```python
from build123d import *

# Parameters (mm, degrees)
SKETCH1_R           = 82.5
BOSS_EXTRUDE1_DEPTH = 13
SKETCH2_R           = 30
CUT_EXTRUDE1_DEPTH  = 118.394633608
SKETCH3_R           = 6.451717482
CUT_EXTRUDE2_DEPTH  = 7.921699
CIRPATTERN1_START   = 5.0783014
CIRPATTERN1_DEPTH   = 7.9216986


# Read off the part's stored shape, not the designer's step: CirPattern1
with BuildPart() as part:
    # Sketch1 → Boss-Extrude1 (new body)
    with BuildSketch(Plane(origin=(0, 0, 0), x_dir=(1, 0, 0), z_dir=(0, 1, 0))):
        with Locations(Location((0, 0, 0), (0, 0, 90))):
            Circle(SKETCH1_R)
    extrude(amount=BOSS_EXTRUDE1_DEPTH)

    # Sketch2 → Cut-Extrude1 (cut, through all)
    with BuildSketch(Plane(origin=(0, 0, 0), x_dir=(1, 0, 0), z_dir=(0, 1, 0))):
        with Locations(Location((0, 0, 0), (0, 0, 90))):
            Circle(SKETCH2_R)
    extrude(amount=CUT_EXTRUDE1_DEPTH, mode=Mode.SUBTRACT)

    # Sketch3 → Cut-Extrude2 (cut)
    with BuildSketch(Plane(origin=(0, 13, 0), x_dir=(1, 0, 0), z_dir=(0, 1, 0))):
        with Locations((-29.738341357, 0)):
            Circle(SKETCH3_R)
    extrude(amount=-CUT_EXTRUDE2_DEPTH, mode=Mode.SUBTRACT)

    # CirPattern1 outline → CirPattern1 (cut)
    with BuildSketch(Plane(origin=(0, 0, 0), x_dir=(1, 0, 0), z_dir=(0, 1, 0)).offset(CIRPATTERN1_START)):
        with BuildLine():
            ThreePointArc((-9.076134205, -28.594121562), (-15, -25.980762114), (-20.225168569, -22.157223571))
            ThreePointArc((-20.225168569, -22.157223571), (-18.095029419, -31.341510319), (-9.076134205, -28.594121562))
        make_face()
        with BuildLine():
            ThreePointArc((-9.076134205, 28.594121562), (-18.095029419, 31.341510319), (-20.225168569, 22.157223571))
            ThreePointArc((-20.225168569, 22.157223571), (-15, 25.980762114), (-9.076134205, 28.594121562))
        make_face()
        with BuildLine():
            ThreePointArc((20.225168569, -22.157223571), (15, -25.980762114), (9.076134205, -28.594121562))
            ThreePointArc((9.076134205, -28.594121562), (18.095029419, -31.341510319), (20.225168569, -22.157223571))
        make_face()
        with BuildLine():
            ThreePointArc((20.225168569, 22.157223571), (18.095029419, 31.341510319), (9.076134205, 28.594121562))
            ThreePointArc((9.076134205, 28.594121562), (15, 25.980762114), (20.225168569, 22.157223571))
        make_face()
        with BuildLine():
            ThreePointArc((29.301302774, 6.436897991), (30, 0), (29.301302774, -6.436897991))
            ThreePointArc((29.301302774, -6.436897991), (36.190058839, 0), (29.301302774, 6.436897991))
        make_face()
    extrude(amount=CIRPATTERN1_DEPTH, mode=Mode.SUBTRACT)


solid = part.part
```
Could you check a few things on this model? Use its own coordinates, in mm. A direction names the side the tool comes from. Round coordinates to 2 decimals unless told otherwise and drop trailing zeros. Write each loop counter-clockwise with the first axis right and the second up, starting at its lowest first coordinate (ties: lowest second). Pieces come first, ordered by that corner, then holes. Notation, with made-up numbers: M 37.5,51.5 L 41.5,51.5 A16 cw 41.5,65.5 Z; hole C 65,-18.5 d4. An arc over 180 degrees is marked long. Answer in a Markdown table with one row per item. Add a question column.
Q1. Imagine slicing it at D-D (z = 48). Please give me the cut outline in (x, y).
Q2. Will these pins go through, and if not, where does the flat tip stop? pin 1 Ø1.5 at (y, z) = (5, -10.5) entering from +X; pin 2 Ø1 at (y, z) = (10, 42) entering from +X; pin 3 Ø8 at (x, z) = (-16.5, -27) entering from +Y.
Q3. If we mould it in two halves opening along X, with no side actions, what happens to faces 3 (the cylindrical face through (80.54, 6.41, 17.88)), 4 (the flat face through (-1, 0, -36)), 5 (the flat face through (-17, 5.078, 28))? For each: +X half, -X half, draft (parallel to the pull), parting line (faces both ways), or undercut.
Q4. Imagine slicing it at A-A (z = 0). Please give me the cut outline in (x, y).
Q5. If I drill on line 1 (X direction, y = 5, z = 0); line 2 (Z direction, x = 1, y = 8); line 3 (X direction, y = 9, z = 27), over which ranges is the centre line in solid material (lowest first)? Write a range as from..to.
Q6. On a 3-axis mill with a long thin cutter (end or side, diameter ignored), from which of +Z, -Z, +X, -X, +Y, -Y can I reach the whole of each face in a straight line? I mean faces 1 (the flat face through (-1, 13, -36)), 2 (the cylindrical face through (18.222, 8.984, -31.266)). Say none if no direction works.
Q7. Imagine slicing it at C-C (y = 7.75). Please give me the cut outline in (x, z), then the cut area to 3 significant figures.
Q8. Imagine slicing it at B-B (x = 0). Please give me the cut outline in (y, z), then the cut area to 4 significant figures.
Values:
| question | item | result |
|---|---|---|
| 1 | outline | M -67.1,0 L 67.1,0 L 67.1,13 L -67.1,13 Z |
| 2 | pin 1 | x = 81.92 |
| 2 | pin 2 | x = 71.3 |
| 2 | pin 3 | y = 5.08 |
| 3 | face 3 | parting line |
| 3 | face 4 | draft |
| 3 | face 5 | undercut |
| 4 | outline | M -82.5,0 L -30,0 L -30,5.08 L -36.19,5.08 L -36.19,13 L -82.5,13 Z; M 30,0 L 82.5,0 L 82.5,13 L 36.19,13 L 36.19,5.08 L 30,5.08 Z |
| 5 | line 1 | -82.5..-30, 30..82.5 |
| 5 | line 2 | -82.49..-29.98, 29.98..82.49 |
| 5 | line 3 | -77.96..-21.2, 21.2..77.96 |
| 6 | face 1 | +Z, -Z, +X, -X, +Y |
| 6 | face 2 | +Y |
| 7 | outline | C 0,0 d165; hole M -29.3,-6.44 A30 ccw -20.23,-22.16 A6.45 ccw long -9.08,-28.59 A30 ccw 9.08,-28.59 A6.45 ccw long 20.23,-22.16 A30 ccw 29.3,-6.44 A6.45 ccw long 29.3,6.44 A30 ccw 20.23,22.16 A6.45 ccw long 9.08,28.59 A30 ccw -9.08,28.59 A6.45 ccw long -20.23,22.16 A30 ccw -29.3,6.44 A6.45 ccw long Z |
| 7 | area | 18,200 mm^2 |
| 8 | outline | M 0,-82.5 L 13,-82.5 L 13,-30 L 0,-30 Z; M 0,30 L 13,30 L 13,82.5 L 0,82.5 Z |
| 8 | area | 1,365 mm^2 |
